Here's the drawing with two shaded views (mm, measured from the low corner). I have some questions. Round coordinates to 2 decimals unless told otherwise and drop trailing zeros. Write each loop counter-clockwise with the first axis right and the second up, starting at its lowest first coordinate (ties: lowest second). Pieces come first, ordered by that corner, then holes. Notation, with made-up numbers: M 1,59 L 5,59 A19 cw 5,91 Z; hole C -9.5,86 d3. An arc over 180 degrees is marked long. Answer as a JSON object with one key per item and string values. Group by question number.
1) Suppose I cut it at A-A, the plane x = 234. Write out the boundary of the cut face in (y, z) (1 decimal).
2) Please list where these lines run through material, in increasing order: L1, parallel to Y at x = 143.5, z = 7.5 (1 decimal); L2, parallel to X at y = 91.5, z = 6.5 (1 decimal). Write a range as [from, to].
3) Suppose I cut it at B-B, the plane z = 1.5. State how many separate pieces and enclosed holes the cut face has, and give its area (3 significant figures).
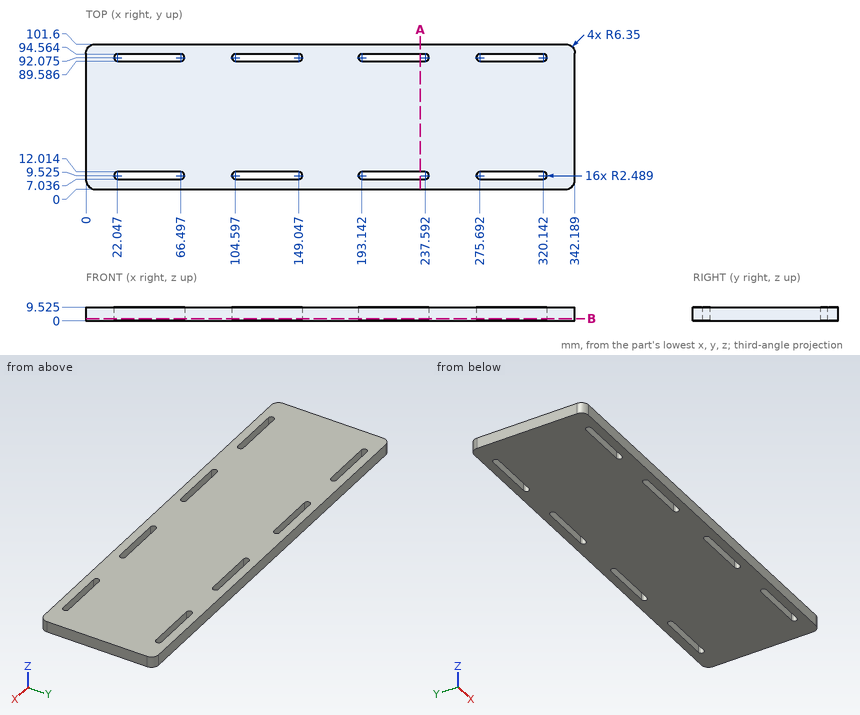
Results:
{
 "1": {"outline": "M 0,0 L 7,0 L 7,9.5 L 0,9.5 Z; M 12,0 L 89.6,0 L 89.6,9.5 L 12,9.5 Z; M 94.6,0 L 101.6,0 L 101.6,9.5 L 94.6,9.5 Z"},
 "2": {"L1": "[0, 7], [12, 89.6], [94.6, 101.6]", "L2": "[0, 19.6], [68.9, 102.2], [151.5, 190.7], [240, 273.3], [322.6, 342.2]"},
 "3": {"separate pieces": "1", "enclosed holes": "8", "area": "32,800 mm^2"}
}
